The model under review builds one solid part; all positions refer to its coordinate system, in mm. A direction names the side the tool comes from. Coordinates: 2 decimals unless noted, no trailing zeros. Write each loop counter-clockwise with the first axis right and the second up, starting at its lowest first coordinate (ties: lowest second). Pieces come first, ordered by that corner, then holes. Notation, with made-up numbers: (38.25, 21) - (47.25, 21) arc R24 ccw to (47.25, 44) - close; hole circle Ø1 at (2, 64.25). An arc over 180 degrees is marked (long way). Put each result on its own line as item: value.
Autodesk Inventor part; units mm, degrees
ref_plane "YZ Plane" through (0, 0, 0) normal (1, 0, 0) x (0, 1, 0)
ref_plane "XZ Plane" through (0, 0, 0) normal (0, 1, 0) x (-1, 0, 0)
ref_plane "XY Plane" through (0, 0, 0) normal (0, 0, 1) x (1, 0, 0)
sketch "スケッチ1" plane through (0, 0, 0) normal (0, 1, 0) x (-1, 0, 0)
  line L0 (0, -13.02) -> (0, 13.02)
  line L1 (-2.4, 0) -> (14.4, 0)
  line L2 (0, -4.8) -> (9.5, -6.65)
  line L3 (9.5, -6.65) -> (9.5, 6.65)
  line L4 (9.5, 6.65) -> (0, 4.8)
  line L5 (0, -9.3) -> (0, -4.8)
  line L6 (0, 4.8) -> (0, 9.3)
  line L7 (2.4, -8.1) -> (11.5, -8.1)
  line L8 (11.5, -8.1) -> (11.5, 8.1)
  line L9 (11.5, 8.1) -> (2.4, 8.1)
  line L10 (2.4, -8.1) -> (0, -9.3)
  line L11 (2.4, 8.1) -> (0, 9.3)
  line L12 (12, -8.1) -> (12, 8.1)
  line L13 (12, 8.1) -> (0, 9.3)
  line L14 (12, -8.1) -> (0, -9.3)
  point P0 (0, 0)
  point P1 (0, 9.3)
  point P2 (0, -9.3)
  dimension "d3" = 13.3
  dimension "d5" = 9.6
  dimension "d14" = 2
  dimension "d63" = 1.2
  dimension "d64" = 18.6
  dimension "d65" = 12
  dimension "d74" = 18.6
  dimension "d75" = 1.2
  dimension "d93" = 9.5
  dimension "d94" = 2.4
extrude "押し出し2" add sketch "スケッチ1" along normal blind 3.2 and the other way blind 5.2 contours L0 L2 L3 L1 L8 L7 L10 | L0 L11 L9 L8 L1 L3 L4
extrude "押し出し1" add sketch "スケッチ1" against normal blind 2 contours L0 L2 L3 L1 L8 L7 L10 | L10 L7 L8 L1 L12 L14 | L1 L8 L9 L11 L13 L12 | L0 L11 L9 L8 L1 L3 L4
chamfer "面取り3" distance 0.5 angle 45 2 edges at (0, -1, 4.8) (0, -1, -4.8)
equation "\"rib\" = 0.5"
equation "\"gap\" = 0.2"
properties part number "StraightRais-215" material "ABS プラスチック"
1. Consider section B-B on x = -5. State the section outline as (y, z) points.
Determined:
outline: (-5.2, -8.1) - (-2, -8.1) - (-2, -8.8) - (0, -8.8) - (0, -8.1) - (3.2, -8.1) - (3.2, -5.77) - (-5.2, -5.77) - close; (-5.2, 5.77) - (3.2, 5.77) - (3.2, 8.1) - (0, 8.1) - (0, 8.8) - (-2, 8.8) - (-2, 8.1) - (-5.2, 8.1) - close
2. For pin 1 Ø1.6 at (x, y) = (-6, -3) entering from -Z; pin 2 Ø2.5 at (x, y) = (-6, -3) entering from +Z (3 decimals); pin 3 Ø2.5 at (x, y) = (-7, 1) entering from -Z (3 decimals), all flat-tipped, find the tip position at first contact; note any pin that passes through.
Determined:
pin 1: stops at z = -8.1
pin 2: stops at z = 8.775
pin 3: stops at z = -8.675
3. Consider section C-C on x = -11. State the section outline as (y, z) points, plus the area to 3 significant figures.
Determined:
outline: (-5.2, -8.1) - (-2, -8.1) - (-2, -8.2) - (0, -8.2) - (0, -8.1) - (3.2, -8.1) - (3.2, 8.1) - (0, 8.1) - (0, 8.2) - (-2, 8.2) - (-2, 8.1) - (-5.2, 8.1) - close
area: 136 mm^2
4. Consider section A-A on z = -7.25. State the section outline as (x, y) points, plus the area to 3 significant figures.
Determined:
outline: (-12, -2) - (-11.5, -2) - (-11.5, -5.2) - (0, -5.2) - (0, 3.2) - (-11.5, 3.2) - (-11.5, 0) - (-12, 0) - close
area: 97.6 mm^2
5. Machinability: for faces 1 (the flat face through (-1.2, 1.6, -8.7)), 2 (the flat face through (-1.2, -3.6, -8.7)), 3 (the flat face through (-11.5, 2, 0)), which of the approach directions +Z, -Z, +X, -X, +Y, -Y give a long, thin tool a straight path to every point of the face, cutting with its end or side? Answer none if there is none.
Determined:
face 1: -Z, -X, +Y
face 2: -Z, -X, -Y
face 3: +Z, -Z, -X, +Y
6. The part is to be moulded in two halves that separate along X. For faces 4 (the flat face through (-5.058, -1.059, 5.785)), 5 (the flat face through (-4.93, -1.06, -5.76)), 6 (the flat face through (-11.7, -2, -0.6)), 7 (the flat face through (-1.2, -3.6, 8.7)), say which applies: +X half, -X half, draft (parallel to the pull), parting line (faces both ways), or undercut.
Determined:
face 4: undercut
face 5: undercut
face 6: draft
face 7: -X half
7. To check wall thickness, follow probe 1 along Z at (x, y) = (-7, -1.75); probe 2 along X at (y, z) = (-4, -1.5); probe 3 along Z at (x, y) = (-6.5, 2). State the ranges of each line that lie inside material, in increasing order.
Determined:
probe 1: z = -8.6 to -6.16, 6.16 to 8.6
probe 2: x = -11.5 to -9.5
probe 3: z = -8.1 to -6.07, 6.07 to 8.1
8. Consider section D-D on z = 6. State the section outline as (x, y) points, plus the area to 3 significant figures.
Determined:
outline: (-12, -2) - (-11.5, -2) - (-11.5, -5.2) - (-9.5, -5.2) - (-9.5, 3.2) - (-11.5, 3.2) - (-11.5, 0) - (-12, 0) - close; (-6.16, -5.2) - (0, -5.2) - (0, 3.2) - (-6.16, 3.2) - close
area: 69.6 mm^2
